For this review, take the finished solid that the model builds, in its own axes (mm). Face numbers are marked on the shaded views. A direction names the side the tool comes from. Give positions to 0.01 mm unless a question says otherwise; leave off trailing zeros. Loops run counter-clockwise (first coordinate to the right, second up) from the corner with the lowest first, then second, coordinate; pieces in that order, holes last. Notation, with made-up numbers: (-4.75, 32.25) -> (46.25, 32.25) arc R18 ccw to (46.25, 60.25) -> close; hole circle Ø1 at (86, -8). An arc over 180 degrees is marked (long way). Answer as CSV lines item,"result". Start each with the question number.
Item 1: Add section C-C on x = 38. State the section outline as (y, z) points.
Item 2: Add section B-B on z = -50. State the section outline as (x, y) points.
Item 3: For L1, parallel to X at y = -62, z = -7; L2, parallel to Y at x = 11, z = -55; L3, parallel to Z at x = 6, y = -44.5, list the stretches that pass through material, from the lowest coordinate up. Write a range as from..to.
Item 4: Machinability: for the marked faces 1 and 2, which of the approach directions +Z, -Z, +X, -X, +Y, -Y give a long, thin tool a straight path to every point of the face, cutting with its end or side? Answer none if there is none.
Item 5: Clearance check with flat-ended pins moving along their axes: P1, Ø6, axis at x = 55, y = -98.5, coming from the +Z side; P2, Ø3, axis at x = 72, y = -59, coming from the +Z side. State where each tip first meets the part, or that it passes through.
Item 6: Add section D-D on y = -95. State the section outline as (x, z) points.
Item 7: Add section A-A on y = -107.5. State the section outline as (x, z) points.
Item 8: The part is to be moulded in two halves that separate along Z. For the marked faces 3, 4, 5 and 6, say which applies: +Z half, -Z half, draft (parallel to the pull), parting line (faces both ways), or undercut.
```python
from build123d import *

# Parameters (mm, degrees)
F1_DEPTH = 25
F2_W     = 10.90179
F2_H     = 55.97822
F2_W_2   = 10.267794
F3_DEPTH = 75
F5_DEPTH = 25
F6_R     = 3.32997
F7_DEPTH = 89.4
F8_W     = 76.124623
F8_H     = 125
F9_DEPTH = 10


with BuildPart() as f1:
    # F0 (on Front) → F1 (new body)
    with BuildSketch(Plane.XZ):
        with BuildLine():
            Line((30.449602, 30.27692), (0, 0))
            Line((0, 0), (38.062312, 0))
            Line((38.062312, 0), (76.124623, 0))
            Line((76.124623, 0), (45.675021, 30.27692))
            ThreePointArc((45.675021, 30.27692), (38.062312, 37.846457), (30.449602, 30.27692))
        make_face()
        Polygon((38.062312, 0), (0, 0), (0, -55.97822), (76.124623, -55.97822), (76.124623, 0), align=None)
    extrude(amount=F1_DEPTH)

    # F2 (on face) → F3 (join)
    with BuildSketch(Plane.XZ.offset(25)):
        with Locations((5.450895, -27.98911)):
            Rectangle(F2_W, F2_H)
        with Locations((70.990726, -27.98911)):
            Rectangle(F2_W_2, F2_H)
    extrude(amount=F3_DEPTH)

    # F4 (on face) → F5 (join)
    with BuildSketch(Plane.XZ.offset(100)):
        with BuildLine():
            Line((30.449602, 30.27692), (0, 0))
            Line((0, 0), (38.062312, 0))
            Line((38.062312, 0), (76.124623, 0))
            Line((76.124623, 0), (45.675021, 30.27692))
            ThreePointArc((45.675021, 30.27692), (38.062312, 37.846457), (30.449602, 30.27692))
        make_face()
        Polygon((38.062312, 0), (0, 0), (0, -55.97822), (76.124623, -55.97822), (76.124623, 0), align=None)
    extrude(amount=F5_DEPTH)

    # F6 (on face) → F7 (join)
    with BuildSketch(Plane(origin=(0, -100, 0), x_dir=(-1, 0, 0), z_dir=(0, 1, 0))):
        with Locations((-38.062312, 30.233625)):
            Circle(F6_R)
    extrude(amount=F7_DEPTH)

    # F8 (on face) → F9 (join)
    with BuildSketch(Plane(origin=(0, 0, -55.97822), x_dir=(1, 0, 0), z_dir=(0, 0, -1))):
        with Locations((38.062311, 62.5)):
            Rectangle(F8_W, F8_H)
    extrude(amount=F9_DEPTH)


solid = f1.part
```
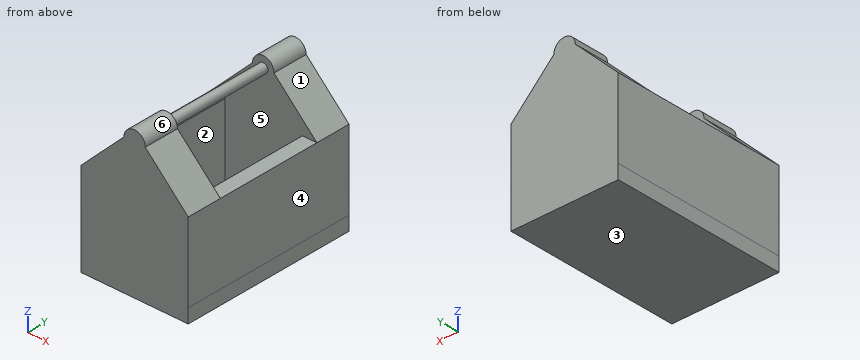
Computed values:
1,outline,"(-125, -65.98) -> (0, -65.98) -> (0, 37.85) -> (-25, 37.85) -> (-25, 33.56) -> (-100, 33.56) -> (-100, 37.85) -> (-125, 37.85) -> close; hole (-100, -55.98) -> (-25, -55.98) -> (-25, 26.9) -> (-100, 26.9) -> close"
2,outline,"(0, -125) -> (76.12, -125) -> (76.12, 0) -> (0, 0) -> close; hole (10.9, -100) -> (65.86, -100) -> (65.86, -25) -> (10.9, -25) -> close"
3,L1,"0..10.9, 65.86..76.12"
3,L2,"-125..-100, -25..0"
3,L3,"-65.98..0"
4,face 1,"+Z, +X, +Y, -Y"
4,face 2,"+Z"
5,P1,"z = 23.59"
5,P2,"z = 0"
6,outline,"(0, -65.98) -> (76.12, -65.98) -> (76.12, 0) -> (65.86, 0) -> (65.86, -55.98) -> (10.9, -55.98) -> (10.9, 0) -> (0, 0) -> close; circle Ø6.66 at (38.06, 30.23)"
7,outline,"(0, -65.98) -> (76.12, -65.98) -> (76.12, 0) -> (45.68, 30.28) arc R7.61 ccw to (30.45, 30.28) -> (0, 0) -> close"
8,face 3,"-Z half"
8,face 4,"draft"
8,face 5,"undercut"
8,face 6,"+Z half"
